Work out the finished part from the listing and answer in its coordinate system (mm). Coordinates: 2 decimals unless noted, no trailing zeros. Write each question's results on one line, items separated by ' | '. Start each with the question number.
Item 1: For a pull along Z with two mould halves and no side action, classify faces 1 (the face through (24, -15, -2)), 2 (the face through (44, -15, -1)) as +Z half, -Z half, draft (parallel to the pull), parting line (faces both ways), or undercut.
Item 2: Consider probe 1 along X at (y, z) = (-13.5, -0.9); probe 2 along X at (y, z) = (-10, -0.9); probe 3 along X at (y, z) = (-17.75, -0.4). Determine where each line is inside the solid, lowest interval first. Write a range as [from, to].
Item 3: Each of these flat-tipped pins is pushed along its axis until it touches: pin 1 Ø1 at (x, z) = (45, -1) entering from +Y; pin 2 Ø0.7 at (x, y) = (44.5, -15.5) entering from +Z. Where does it stop, or does it pass through?
from build123d import *

# Parameters (mm, degrees)
EXTRUDE002_DEPTH = 5
EXTRUDE001_DEPTH = 2
EXTRUDE_DEPTH    = 2


with BuildPart() as obj1:
    # path4171 → Extrude002 (new body)
    with BuildSketch(Plane(origin=(6.373784, -15.136707, 0), x_dir=(0, 1, 0), z_dir=(0, 0, 1))):
        with BuildLine():
            add(Edge.make_bspline(
                [(-5.911478, 1.599036), (-5.911478, -1.599036)],
                knots=[0, 0, 11.33175, 11.33175], degree=1))
            add(Edge.make_bspline(
                [(-5.911478, -1.599036), (5.911478, -1.599036)],
                knots=[0, 0, 41.89236, 41.89236], degree=1))
            add(Edge.make_bspline(
                [(5.911478, -1.599036), (5.911478, 1.599036)],
                knots=[0, 0, 11.33175, 11.33175], degree=1))
            add(Edge.make_bspline(
                [(5.911478, 1.599036), (-5.911478, 1.599036)],
                knots=[0, 0, 41.89236, 41.89236], degree=1))
        make_face()
    extrude(amount=EXTRUDE002_DEPTH)


with BuildPart() as obj1_1:
    # Extrude002 placement: moved
    add(obj1.part.moved(Location((0, 0, -3))))


with BuildPart() as obj2:
    # path4175 → Extrude001 (new body)
    with BuildSketch(Plane(origin=(45.980416, -15.300068, 0), x_dir=(0, -1, 0), z_dir=(0, 0, -1))):
        with BuildLine():
            add(Edge.make_bspline(
                [(-0.66988, 20.181412), (-0.616291, -20.181412)],
                knots=[0, 0, 143.018006, 143.018006], degree=1))
            add(Edge.make_bspline(
                [(-0.616291, -20.181412), (0.509109, -18.969959)],
                knots=[0, 0, 5.858947, 5.858947], degree=1))
            add(Edge.make_bspline(
                [(0.509109, -18.969959), (0.66988, 16.950874)],
                knots=[0, 0, 127.279815, 127.279815], degree=1))
            add(Edge.make_bspline(
                [(0.66988, 16.950874), (-0.66988, 20.181412)],
                knots=[0, 0, 12.392123, 12.392123], degree=1))
        make_face()
    extrude(amount=EXTRUDE001_DEPTH)


with BuildPart() as obj2_1:
    # Extrude001 placement: moved
    add(obj2.part.moved(Location((0, 0, 1))))


with BuildPart() as obj3:
    # path4167 → Extrude (new body)
    with BuildSketch(Plane(origin=(31.691849, -15.004078, 0), x_dir=(0, -1, 0), z_dir=(0, 0, -1))):
        with BuildLine():
            add(Edge.make_bspline(
                [(9.606149, 31.409626), (-10.174564, 31.409626)],
                knots=[0, 0, 70.08914, 70.08914], degree=1))
            add(Edge.make_bspline(
                [(-10.174564, 31.409626), (-14.721856, 26.840954)],
                knots=[0, 0, 22.840078, 22.840078], degree=1))
            add(Edge.make_bspline(
                [(-14.721856, 26.840954), (-14.721856, 9.479997)],
                knots=[0, 0, 61.5152, 61.5152], degree=1))
            add(Edge.make_bspline(
                [(-14.721856, 9.479997), (-10.212458, 4.949393)],
                knots=[0, 0, 22.649752, 22.649752], degree=1))
            add(Edge.make_bspline(
                [(-10.212458, 4.949393), (-5.627273, 4.949393)],
                knots=[0, 0, 16.24672, 16.24672], degree=1))
            add(Edge.make_bspline(
                [(-5.627273, 4.949393), (-8.905112, 1.656139)],
                knots=[0, 0, 16.463895, 16.463895], degree=1))
            add(Edge.make_bspline(
                [(-8.905112, 1.656139), (-8.905112, -0.494942)],
                knots=[0, 0, 7.62194, 7.62194], degree=1))
            add(Edge.make_bspline(
                [(-8.905112, -0.494942), (-4.490451, -0.494942)],
                knots=[0, 0, 15.6425, 15.6425], degree=1))
            add(Edge.make_bspline(
                [(-4.490451, -0.494942), (-4.490451, -27.06939)],
                knots=[0, 0, 94.16143, 94.16143], degree=1))
            add(Edge.make_bspline(
                [(-4.490451, -27.06939), (-1.913652, -31.409626)],
                knots=[0, 0, 17.884943, 17.884943], degree=1))
            add(Edge.make_bspline(
                [(-1.913652, -31.409626), (-0.625254, -31.409626)],
                knots=[0, 0, 4.56519, 4.56519], degree=1))
            add(Edge.make_bspline(
                [(-0.625254, -31.409626), (4.300981, -26.155653)],
                knots=[0, 0, 25.519687, 25.519687], degree=1))
            add(Edge.make_bspline(
                [(4.300981, -26.155653), (4.376766, -22.957582)],
                knots=[0, 0, 11.334931, 11.334931], degree=1))
            add(Edge.make_bspline(
                [(4.376766, -22.957582), (2.330485, -20.21638)],
                knots=[0, 0, 12.120727, 12.120727], degree=1))
            add(Edge.make_bspline(
                [(2.330485, -20.21638), (5.665167, -17.018305)],
                knots=[0, 0, 16.371375, 16.371375], degree=1))
            add(Edge.make_bspline(
                [(5.665167, -17.018305), (5.665167, -14.581683)],
                knots=[0, 0, 8.6337, 8.6337], degree=1))
            add(Edge.make_bspline(
                [(5.665167, -14.581683), (2.557849, -11.155178)],
                knots=[0, 0, 16.389992, 16.389992], degree=1))
            add(Edge.make_bspline(
                [(2.557849, -11.155178), (6.119891, -7.72867)],
                knots=[0, 0, 17.513081, 17.513081], degree=1))
            add(Edge.make_bspline(
                [(6.119891, -7.72867), (3.543095, -4.682891)],
                knots=[0, 0, 14.136262, 14.136262], degree=1))
            add(Edge.make_bspline(
                [(3.543095, -4.682891), (3.543095, -0.799519)],
                knots=[0, 0, 13.75998, 13.75998], degree=1))
            add(Edge.make_bspline(
                [(3.543095, -0.799519), (8.92406, -0.799519)],
                knots=[0, 0, 19.06641, 19.06641], degree=1))
            add(Edge.make_bspline(
                [(8.92406, -0.799519), (8.92406, 0.190362)],
                knots=[0, 0, 3.50745, 3.50745], degree=1))
            add(Edge.make_bspline(
                [(8.92406, 0.190362), (6.498837, 4.530598)],
                knots=[0, 0, 17.616815, 17.616815], degree=1))
            add(Edge.make_bspline(
                [(6.498837, 4.530598), (10.818765, 4.530598)],
                knots=[0, 0, 15.30683, 15.30683], degree=1))
            add(Edge.make_bspline(
                [(10.818765, 4.530598), (14.721856, 8.452045)],
                knots=[0, 0, 19.604406, 19.604406], degree=1))
            add(Edge.make_bspline(
                [(14.721856, 8.452045), (14.721856, 26.9171)],
                knots=[0, 0, 65.42736, 65.42736], degree=1))
            add(Edge.make_bspline(
                [(14.721856, 26.9171), (9.606149, 31.409626)],
                knots=[0, 0, 24.123975, 24.123975], degree=1))
        make_face()
    extrude(amount=EXTRUDE_DEPTH)

    # Cut: cut obj2
    add(obj2_1.part, mode=Mode.SUBTRACT)

    # Cut001: cut obj1
    add(obj1_1.part, mode=Mode.SUBTRACT)


solid = obj3.part
Answer key:
1) face 1: -Z half | face 2: +Z half
2) probe 1: x = [0.28, 4.77], [7.97, 63.1] | probe 2: x = [0.28, 4.77], [7.97, 32.19] | probe 3: x = [0.28, 4.77], [7.97, 42.67], [43.05, 51.51], [52.46, 59.51]
3) pin 1: stops at y = -10.51 | pin 2: stops at z = -1
